Can you work these out from the model? Positions are in its coordinate system, mm. A direction names the side the tool comes from. Round coordinates to 2 decimals unless told otherwise and drop trailing zeros. Order: outer loops, then holes, each group sorted by start corner. A loop starts at its lowest first (then second) coordinate and runs counter-clockwise, first axis right, second up. Notation, with made-up numbers: (46, 18) - (90, 18) arc R23 ccw to (90, 32) - close; hole circle Ø8 at (88, 49). An arc over 180 degrees is marked (long way). Write item = value, one per line.
from build123d import *

# Parameters (mm, degrees)
ESQUISSE1_W         = 54
ESQUISSE1_H         = 40
BOSS_EXTRU_9_DEPTH  = 2
ESQUISSE1_14_W      = 54
ESQUISSE1_14_H      = 3
ESQUISSE1_14_W_2    = 3
BOSS_EXTRU_10_DEPTH = 35
CONG_14_R           = 4
ESQUISSE1_18_W      = 10
ESQUISSE1_18_H      = 2
ESQUISSE1_18_H_2    = 20
BOSS_EXTRU_12_DEPTH = 2
ESQUISSE1_20_W      = 10
ESQUISSE1_20_H      = 2
BOSS_EXTRU_13_DEPTH = 2
BOSS_EXTRU_15_START = -2
ESQUISSE9_W         = 10
ESQUISSE9_H         = 24
BOSS_EXTRU_15_DEPTH = 2
CONG_15_R           = 2


with BuildPart() as part:
    # Esquisse1 → Boss.-Extru.9 (new body)
    with BuildSketch(Plane(origin=(0, 0, 0), x_dir=(1, 0, 0), z_dir=(0, 1, 0))):
        with Locations((30, 23)):
            Rectangle(ESQUISSE1_W, ESQUISSE1_H)
        Polygon((35, 33), (35, 13), (35, 11), (25, 11), (25, 13), (25, 33), (25, 35), (35, 35), align=None, mode=Mode.SUBTRACT)
    extrude(amount=BOSS_EXTRU_9_DEPTH)

    # Esquisse1_14 → Boss.-Extru.10 (add)
    with BuildSketch(Plane(origin=(0, 0, 0), x_dir=(1, 0, 0), z_dir=(0, 1, 0))):
        Polygon((60, 46), (57, 46), (57, 43), (57, 3), (57, 0), (60, 0), align=None)
        with Locations((30, 44.5)):
            Rectangle(ESQUISSE1_14_W, ESQUISSE1_14_H)
        with Locations((1.5, 44.5)):
            Rectangle(ESQUISSE1_14_W_2, ESQUISSE1_14_H)
        Polygon((3, 43), (0, 43), (0, 0), (3, 0), (3, 3), align=None)
        with Locations((30, 1.5)):
            Rectangle(ESQUISSE1_14_W, ESQUISSE1_14_H)
    extrude(amount=BOSS_EXTRU_10_DEPTH)

    # Cong_14
    cong_14_edges = [part.edges().sort_by_distance(p)[0] for p in [
        (60, 17.5, -46),
        (0, 17.5, -46),
        (0, 17.5, 0),
        (60, 17.5, 0),
    ]]
    fillet(cong_14_edges, radius=CONG_14_R)

    # Esquisse1_18 → Boss.-Extru.12 (add)
    with BuildSketch(Plane(origin=(0, 0, 0), x_dir=(1, 0, 0), z_dir=(0, 1, 0))):
        with Locations((30, 34)):
            Rectangle(ESQUISSE1_18_W, ESQUISSE1_18_H)
        with Locations((30, 23)):
            Rectangle(ESQUISSE1_18_W, ESQUISSE1_18_H_2)
        with Locations((30, 12)):
            Rectangle(ESQUISSE1_18_W, ESQUISSE1_18_H)
    extrude(amount=BOSS_EXTRU_12_DEPTH)

    # Esquisse1_20 → Boss.-Extru.13 (add)
    with BuildSketch(Plane(origin=(0, 0, 0), x_dir=(1, 0, 0), z_dir=(0, 1, 0))):
        with Locations((30, 34)):
            Rectangle(ESQUISSE1_20_W, ESQUISSE1_20_H)
        with Locations((30, 12)):
            Rectangle(ESQUISSE1_20_W, ESQUISSE1_20_H)
    extrude(amount=-BOSS_EXTRU_13_DEPTH)

    # Esquisse9 → Boss.-Extru.15 (add)
    with BuildSketch(Plane(origin=(0, 0, 0), x_dir=(1, 0, 0), z_dir=(0, 1, 0)).offset(BOSS_EXTRU_15_START)):
        with Locations((30, 23)):
            Rectangle(ESQUISSE9_W, ESQUISSE9_H)
    extrude(amount=-BOSS_EXTRU_15_DEPTH)

    # Cong_15
    cong_15_edges = [part.edges().sort_by_distance(p)[0] for p in [
        (30, -4, -35),
        (30, -4, -11),
    ]]
    fillet(cong_15_edges, radius=CONG_15_R)


solid = part.part
(1) If I drill on line 1 (X direction, y = 11.5, z = -18); line 2 (Y direction, x = 32.5, z = -22); line 3 (Z direction, x = 7.5, y = 11), over which ranges is the centre line in solid material (lowest first)? Write a range as from..to.
Computed:
line_1 = 0..3, 57..60
line_2 = -4..-2, 0..2
line_3 = -46..-43, -3..0
(2) If we section it at B-B (x = 11): Write out the boundary of the cut face in (y, z).
Computed:
outline = (0, -46) - (35, -46) - (35, -43) - (2, -43) - (2, -3) - (35, -3) - (35, 0) - (0, 0) - close
(3) If we section it at A-A (z = -21): Write out the boundary of the cut face in (x, y), plus the area to 3 significant figures.
Computed:
outline = (0, 0) - (60, 0) - (60, 35) - (57, 35) - (57, 2) - (3, 2) - (3, 35) - (0, 35) - close; (25, -4) - (35, -4) - (35, -2) - (25, -2) - close
area = 338 mm^2
(4) Will these pins go through, and if not, where does the flat tip stop? P1, Ø4, axis at x = 45, z = -32.5, coming from the +Y side; P2, Ø4.5, axis at y = -3, z = -26, coming from the -X side; P3, Ø1.2, axis at y = -3, z = -25, coming from the +X side.
Computed:
P1 = 2
P2 = 25
P3 = 35
(5) Thinking about a two-plate mould opening in Z: for faces 4 (the face through (1.203, 17.745, -44.859)), 5 (the face through (58.859, 17.745, -1.203)), 6 (the face through (30, 18, -3)), 7 (the face through (30, -1, -13)), which applies, +Z half, -Z half, draft (parallel to the pull), parting line (faces both ways), or undercut?
Computed:
face_4 = -Z half
face_5 = +Z half
face_6 = undercut
face_7 = undercut
(6) On a 3-axis mill with a long thin cutter (end or side, diameter ignored), from which of +Z, -Z, +X, -X, +Y, -Y can I reach the whole of each face in a straight line? I mean faces 1 (the face through (25, -3, -23)), 2 (the face through (57, 18, -23)), 3 (the face through (35, -3, -23)). Say none if no direction works.
Computed:
face_1 = +Z, -Z, -X, -Y
face_2 = +Y
face_3 = +Z, -Z, +X, -Y
(7) If we section it at C-C (y = 28): Write out the boundary of the cut face in (x, z).
Computed:
outline = (0, -42) arc R4 ccw to (4, -46) - (56, -46) arc R4 ccw to (60, -42) - (60, -4) arc R4 ccw to (56, 0) - (4, 0) arc R4 ccw to (0, -4) - close; hole (3, -43) - (57, -43) - (57, -3) - (3, -3) - close
(8) If we section it at D-D (z = -10): Write out the boundary of the cut face in (x, y).
Computed:
outline = (0, 0) - (60, 0) - (60, 35) - (57, 35) - (57, 2) - (3, 2) - (3, 35) - (0, 35) - close
